The model under review builds one solid part; all positions refer to its coordinate system, in mm. A direction names the side the tool comes from. Round coordinates to 2 decimals unless told otherwise and drop trailing zeros. Write each loop counter-clockwise with the first axis right and the second up, starting at its lowest first coordinate (ties: lowest second). Pieces come first, ordered by that corner, then holes. Notation, with made-up numbers: (30.5, 36.5) - (43.5, 36.5) arc R25 cw to (43.5, 60.5) - close; hole circle Ø10 at (11.5, 19.5). An arc over 180 degrees is marked (long way). Use one line per item in the form item = value.
from build123d import *

# Parameters (mm, degrees)
SKETCH1_W         = 40
SKETCH1_H         = 30
PERFBOARD_DEPTH   = 1.6
DIP8_SOCKET_START = 1.6
SKETCH2_W         = 10.2
SKETCH2_H         = 7.6
DIP8_SOCKET_DEPTH = 3
CA3140_START      = 4.6
SKETCH3_W         = 9.3
SKETCH3_H         = 6.35
CA3140_DEPTH      = 3.3
HEADER_START      = 1.6
SKETCH4_W         = 2.5
SKETCH4_H         = 7.6
HEADER_DEPTH      = 8.5


with BuildPart() as part:
    # Sketch1 → Perfboard (new body)
    with BuildSketch(Plane(origin=(0, 0, 0), x_dir=(1, 0, 0), z_dir=(0, 1, 0))):
        Rectangle(SKETCH1_W, SKETCH1_H)
    extrude(amount=PERFBOARD_DEPTH)

    # Sketch2 → DIP8_Socket (add)
    with BuildSketch(Plane(origin=(0, 0, 0), x_dir=(1, 0, 0), z_dir=(0, 1, 0)).offset(DIP8_SOCKET_START)):
        Rectangle(SKETCH2_W, SKETCH2_H)
    extrude(amount=DIP8_SOCKET_DEPTH)

    # Sketch3 → CA3140 (add)
    with BuildSketch(Plane(origin=(0, 0, 0), x_dir=(1, 0, 0), z_dir=(0, 1, 0)).offset(CA3140_START)):
        Rectangle(SKETCH3_W, SKETCH3_H)
    extrude(amount=CA3140_DEPTH)

    # Sketch4 → Header (add)
    with BuildSketch(Plane(origin=(0, 0, 0), x_dir=(1, 0, 0), z_dir=(0, 1, 0)).offset(HEADER_START)):
        with Locations((16, 0)):
            Rectangle(SKETCH4_W, SKETCH4_H)
    extrude(amount=HEADER_DEPTH)


solid = part.part
(1) To check wall thickness, follow L1, parallel to X at y = 5.75, z = 2.25; L2, parallel to Y at x = -17.5, z = -2; L3, parallel to Y at x = -1, z = 3.25. State the ranges of each line that lie inside material, in increasing order.
Geometry results:
L1 = -4.65 to 4.65, 14.75 to 17.25
L2 = 0 to 1.6
L3 = 0 to 4.6
(2) Add section D-D on z = 11. Write out the cut boundary in (x, y), then the cut area to 3 significant figures.
Geometry results:
outline = (-20, 0) - (20, 0) - (20, 1.6) - (-20, 1.6) - close
area = 64.0 mm2
(3) Add section B-B on x = -4. Write out the cut boundary in (y, z) (3 decimals).
Geometry results:
outline = (0, -15) - (1.6, -15) - (1.6, -3.8) - (4.6, -3.8) - (4.6, -3.175) - (7.9, -3.175) - (7.9, 3.175) - (4.6, 3.175) - (4.6, 3.8) - (1.6, 3.8) - (1.6, 15) - (0, 15) - close
(4) Machinability: for faces 1 (the flat face through (17.25, 6, 0)), 2 (the flat face through (16, 6, -3.8)), 3 (the flat face through (14.75, 6, 0)), 4 (the flat face through (0, 6, 3.175)), which of the approach directions +Z, -Z, +X, -X, +Y, -Y give a long, thin tool a straight path to every point of the face, cutting with its end or side? Answer none if there is none.
Geometry results:
face_1 = +Z, -Z, +X, +Y
face_2 = -Z, +X, -X, +Y
face_3 = +Z, -Z, +Y
face_4 = +Z, -X, +Y
(5) Add section A-A on y = 3. Write out the cut boundary in (x, z), then the cut area to 3 significant figures.
Geometry results:
outline = (-5.1, -3.8) - (5.1, -3.8) - (5.1, 3.8) - (-5.1, 3.8) - close; (14.75, -3.8) - (17.25, -3.8) - (17.25, 3.8) - (14.75, 3.8) - close
area = 96.5 mm2
(6) Insertion check: P1, Ø2.5, axis at x = -2.5, z = 1, coming from the +Y side; P2, Ø2.5, axis at x = 0.5, y = 6.5, coming from the -Z side (3 decimals); P3, Ø1.5, axis at y = 3, z = 12, coming from the -X side; P4, Ø3.5, axis at x = 1.5, y = 3.5, coming from the +Z side. Each pin has a flat end and moves straight along its axis. Give the tip position at first contact, or say it passes through.
Geometry results:
P1 = 7.9
P2 = -3.175
P3 = through
P4 = 3.8
(7) Add section C-C on y = 7.25. Write out the cut boundary in (x, z) (3 decimals).
Geometry results:
outline = (-4.65, -3.175) - (4.65, -3.175) - (4.65, 3.175) - (-4.65, 3.175) - close; (14.75, -3.8) - (17.25, -3.8) - (17.25, 3.8) - (14.75, 3.8) - close
